Input: part model. Units: mm. Frame: model coordinates. A direction names the side the tool comes from. Give positions to 0.01 mm unless a question says otherwise; leave off trailing zeros. Loops run counter-clockwise (first coordinate to the right, second up) from the corner with the lowest first, then second, coordinate; pieces in that order, holes last. Notation, with made-up numbers: M 27.25,83 L 44.25,83 A20 ccw 44.25,119 Z; hole C -22.5,-4.75 d4. An arc over 180 degrees is marked long. Answer as a JSON object with one key per item and string values. Group by question number.
1) Section query C-C on z = 184. Return loops of the section in (x, y).
2) Ray query, L1, parallel to Z at x = 0, y = 12; L2, parallel to X at y = 24, z = 156; L3, parallel to X at y = 12, z = 98. Return the intervals inside material, ascending.
3) Access query for faces 1 (the flat face through (0, 5, 26)), 2 (the flat face through (-32, 0, 75.019)), 3 (the flat face through (-32, 9, 84)), 4 (the flat face through (-77.885, -19.551, 82.357)). Directions: +Z, -Z, +X, -X, +Y, -Y. A direction counts if a zero-diameter tool reaches every point of the face in a straight line with its end or side. Return the directions, or none.
4) First-contact query: P1, Ø24, axis at x = -5.5, y = 0, coming from the +Z side; P2, Ø20, axis at x = -31.5, y = 2.5, coming from the -Z side; P3, Ø20, axis at x = 39.5, z = 85, coming from the -Y side. Flat tips, straight axial feed; report the tip coordinate or a pass-through.
5) Section query D-D on z = 82. Return loops of the section in (x, y), plus the area to 3 significant figures.
6) Section query B-B on z = 118.5. Return loops of the section in (x, y), plus the area to 3 significant figures.
7) Section query A-A on x = 63.5. Return loops of the section in (y, z), plus the area to 3 significant figures.
8) Draft query along Z for faces 5 (the cylindrical face through (-2.538, -12.605, 31.165)), 6 (the cylindrical face through (5.513, 17.465, 17.639)), 7 (the flat face through (-4, -20, 31)), 8 (the flat face through (-77.9, 40.4, 170.1)). Return one class per face: +Z half, -Z half, draft (parallel to the pull), parting line (faces both ways), or undercut.
from build123d import *

# Parameters (mm, degrees)
SKETCH_2_W               = 30
SKETCH_2_H               = 30
EXTRUDE_1_DEPTH          = 100
SKETCH_3_W               = 18
SKETCH_3_H               = 18
EXTRUDE_2_DEPTH          = 35
PATTERN_CIRCULAR_1_COUNT = 2
SKETCH_4_R               = 10.254249717
EXTRUDE_4_DEPTH          = 5
SKETCH_5_R               = 5.5
CUT_EXTRUDE_2_DEPTH      = 15
PATTERN_CIRCULAR_3_COUNT = 2
PATTERN_CIRCULAR_4_COUNT = 2
EXTRUDE_5_DEPTH          = 55
PATTERN_LINEAR_1_COUNT   = 2
PATTERN_LINEAR_1_PITCH   = 155
SKETCH_7_W               = 55
SKETCH_7_H               = 5
EXTRUDE_6_DEPTH          = 90


with BuildPart() as part:
    # 草图2 → 凸台-拉伸1 (new body)
    with BuildSketch(Plane.XY):
        Rectangle(SKETCH_2_W, SKETCH_2_H)
    extrude(amount=EXTRUDE_1_DEPTH)

    # 草图3 → 凸台-拉伸2 (add)
    with BuildSketch(Plane(origin=(15, 0, 0), x_dir=(0, 0, -1), z_dir=(1, 0, 0))):
        with Locations((-84.019000904, 0)):
            Rectangle(SKETCH_3_W, SKETCH_3_H)
    extrude_2 = extrude(amount=EXTRUDE_2_DEPTH)

    # 阵列(圆周)1: 凸台-拉伸2 ×2 about axis
    pattern_circular_1_axis = Axis((0, 0, 0), (0, 0, 1))
    for i in range(1, PATTERN_CIRCULAR_1_COUNT):
        add(extrude_2.rotate(pattern_circular_1_axis, i * 360 / PATTERN_CIRCULAR_1_COUNT))

    # 草图4 → 凸台-拉伸4 (add)
    with BuildSketch(Plane(origin=(0, 15, 0), x_dir=(1, 0, 0), z_dir=(0, 1, 0))):
        with Locations((0, -26.28538531)):
            Circle(SKETCH_4_R)
    extrude_4 = extrude(amount=EXTRUDE_4_DEPTH)

    # 草图5 → 切除-拉伸2 (cut)
    with BuildSketch(Plane(origin=(0, 20, 0), x_dir=(1, 0, 0), z_dir=(0, 1, 0))):
        with Locations((0, -26.28538531)):
            Circle(SKETCH_5_R)
    cut_extrude_2 = extrude(amount=-CUT_EXTRUDE_2_DEPTH, mode=Mode.SUBTRACT)

    # 阵列(圆周)3: 凸台-拉伸4 ×2 about axis
    pattern_circular_3_axis = Axis((0, 0, 100), (0, 0, -1))
    for i in range(1, PATTERN_CIRCULAR_3_COUNT):
        add(extrude_4.rotate(pattern_circular_3_axis, i * 360 / PATTERN_CIRCULAR_3_COUNT))

    # 阵列(圆周)4: 切除-拉伸2 ×2 about axis
    pattern_circular_4_axis = Axis((0, 0, 100), (0, 0, -1))
    for i in range(1, PATTERN_CIRCULAR_4_COUNT):
        add(cut_extrude_2.rotate(pattern_circular_4_axis, i * 360 / PATTERN_CIRCULAR_4_COUNT), mode=Mode.SUBTRACT)

    # 草图6 → 凸台-拉伸5 (add)
    with BuildSketch(Plane(origin=(50, 0, 0), x_dir=(0, 0, -1), z_dir=(1, 0, 0))):
        Polygon((-64.431978069, -1.626144526), (-106.85838494, 40.800262345), (-142.213724, 5.444923286), (-99.787317129, -36.981483585), align=None)
    extrude_5 = extrude(amount=EXTRUDE_5_DEPTH)

    # 阵列(线性)1: 凸台-拉伸5 ×2
    with Locations(*[(-i * PATTERN_LINEAR_1_PITCH, 0, 0) for i in range(1, PATTERN_LINEAR_1_COUNT)]):
        add(extrude_5)

    # 草图7 → 凸台-拉伸6 (add)
    with BuildSketch(Plane(origin=(0, 73.829323643, 73.829323643), x_dir=(1, 0, 0), z_dir=(0, 0.707106781, 0.707106781))):
        with Locations((77.5, -94.21014644)):
            Rectangle(SKETCH_7_W, SKETCH_7_H)
        with Locations((77.5, -49.21014644)):
            Rectangle(SKETCH_7_W, SKETCH_7_H)
        with Locations((-77.5, -94.21014644)):
            Rectangle(SKETCH_7_W, SKETCH_7_H)
        with Locations((-77.5, -49.21014644)):
            Rectangle(SKETCH_7_W, SKETCH_7_H)
    extrude(amount=EXTRUDE_6_DEPTH)


solid = part.part
Output:
{
 "1": {"outline": "M -105,47.23 L -50,47.23 L -50,54.3 L -105,54.3 Z; M 50,47.23 L 105,47.23 L 105,54.3 L 50,54.3 Z"},
 "2": {"L1": "z = 0 to 20.79, 31.79 to 100", "L2": "x = -105 to -50, 50 to 105", "L3": "x = -105 to -50, -15 to 15, 50 to 105"},
 "3": {"face 1": "+Y", "face 2": "-Z, +Y, -Y", "face 3": "+Z, -Z, +Y", "face 4": "-Z, -X, -Y"},
 "4": {"P1": "stops at z = 100", "P2": "stops at z = 75.02", "P3": "stops at y = -9"},
 "5": {"outline": "M -105,-19.19 L -50,-19.19 L -50,-9 L -15,-9 L -15,-15 L 15,-15 L 15,-9 L 50,-9 L 50,-19.19 L 105,-19.19 L 105,15.94 L 50,15.94 L 50,9 L 15,9 L 15,15 L -15,15 L -15,9 L -50,9 L -50,15.94 L -105,15.94 Z", "area": "6,020 mm^2"},
 "6": {"outline": "M -105,-18.27 L -50,-18.27 L -50,29.16 L -105,29.16 Z; M -105,45.37 L -50,45.37 L -50,52.44 L -105,52.44 Z; M 50,-18.27 L 105,-18.27 L 105,29.16 L 50,29.16 Z; M 50,45.37 L 105,45.37 L 105,52.44 L 50,52.44 Z", "area": "5,990 mm^2"},
 "7": {"outline": "M -36.98,99.79 L -1.63,64.43 L 104.44,170.5 L 100.9,174.03 L 37.26,110.39 L 8.98,138.68 L 72.62,202.32 L 69.08,205.85 Z", "area": "3,900 mm^2"},
 "8": {"face 5": "undercut", "face 6": "parting line", "face 7": "draft", "face 8": "undercut"}
}
